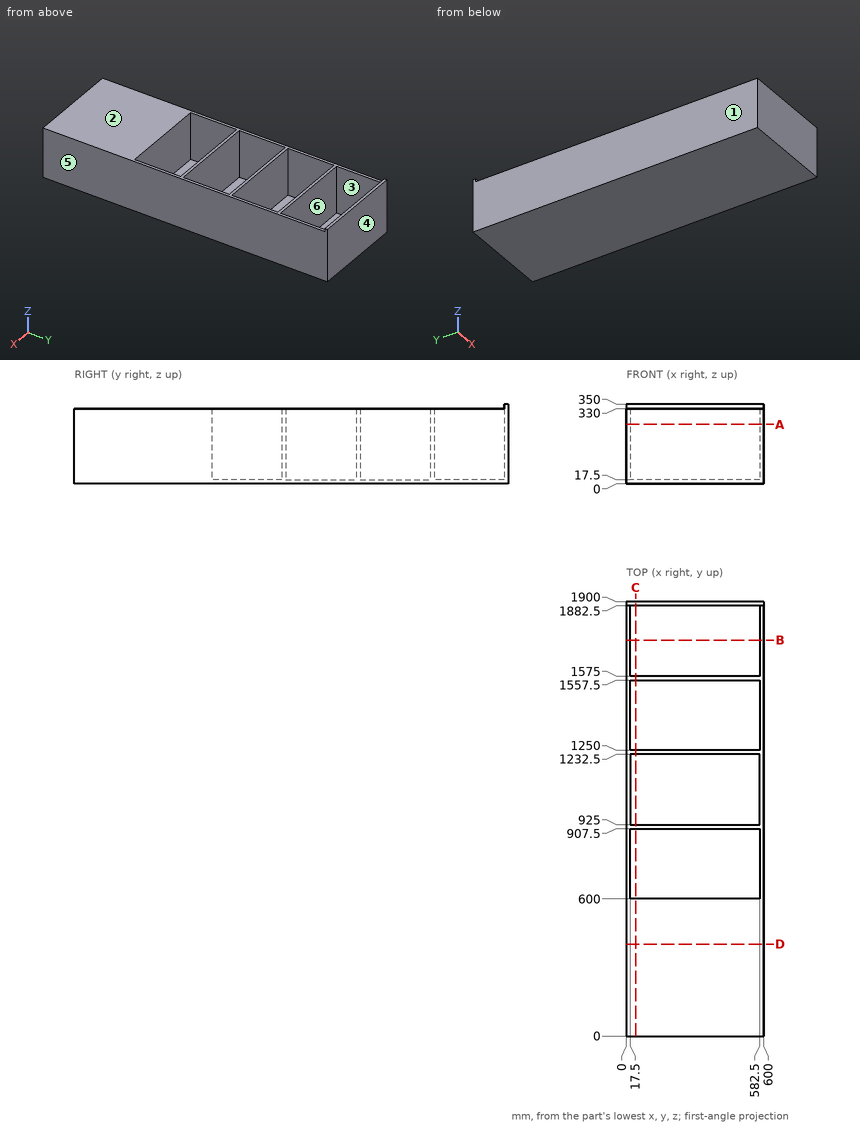
Could you check a few things on this drawing? It's one solid part, dimensions in mm from its lowest x, y, z. A direction names the side the tool comes from. Round coordinates to 2 decimals unless told otherwise and drop trailing zeros. Loops run counter-clockwise (first coordinate to the right, second up) from the corner with the lowest first, then second, coordinate; pieces in that order, holes last. Notation, with made-up numbers: (21.5, 48) -> (76.5, 48) arc R11 cw to (76.5, 59) -> close; hole circle Ø1 at (-30, 63). An arc over 180 degrees is marked (long way). One line per item, written item: value. Start each with the question number.
1. If we section it at C-C, the plane x = 40: Write out the boundary of the cut face in (y, z), then the cut area to 3 significant figures.
2. If we section it at A-A, the plane z = 260.5: Write out the boundary of the cut face in (x, y), then the cut area to 3 significant figures.
3. If we section it at D-D, the plane y = 402: Write out the boundary of the cut face in (x, z), then the cut area to 3 significant figures.
4. For pin 1 (5 mm diameter, centred on x = 304.5, y = 1248, fed in from +Z), with a flat end and sliding along its axis, tell me the tip position at first contact or that it passes through.
5. If I drill on probe 1 along Y at (x, z) = (460.5, 40.5); probe 2 along X at (y, z) = (928, 70.5); probe 3 along Z at (x, y) = (121, 1208), over which ranges is the centre line in solid material (lowest first)?
6. If we mould it in two halves opening along Y, with no side actions, what happens to the marked faces 4, 5 and 6? For each: pulls with the +Y half, pulls with the -Y half, needs draft (parallel to the pull), parting line crosses it, or undercut.
7. If we section it at B-B, the plane y = 1733: Write out the boundary of the cut face in (x, z), then the cut area to 3 significant figures.
8. For the marked faces 1, 2 and 3, which set-ups out of +Z, -Z, +X, -X, +Y, -Y let a thin tool reach every point of the face, with its end or its side?
Calculated:
1. outline: (0, 0) -> (1900, 0) -> (1900, 350) -> (1882.5, 350) -> (1882.5, 17.5) -> (1575, 17.5) -> (1575, 330) -> (1557.5, 330) -> (1557.5, 17.5) -> (1250, 17.5) -> (1250, 330) -> (1232.5, 330) -> (1232.5, 17.5) -> (925, 17.5) -> (925, 330) -> (907.5, 330) -> (907.5, 17.5) -> (600, 17.5) -> (600, 330) -> (0, 330) -> close
1. area: 243,000 mm²
2. outline: (0, 0) -> (600, 0) -> (600, 1900) -> (0, 1900) -> close; hole (17.5, 600) -> (582.5, 600) -> (582.5, 907.5) -> (17.5, 907.5) -> close; hole (17.5, 925) -> (582.5, 925) -> (582.5, 1232.5) -> (17.5, 1232.5) -> close; hole (17.5, 1250) -> (582.5, 1250) -> (582.5, 1557.5) -> (17.5, 1557.5) -> close; hole (17.5, 1575) -> (582.5, 1575) -> (582.5, 1882.5) -> (17.5, 1882.5) -> close
2. area: 445,000 mm²
3. outline: (0, 0) -> (600, 0) -> (600, 330) -> (0, 330) -> close
3. area: 198,000 mm²
4. pin 1: stops at z = 330
5. probe 1: y = 0 to 600, 907.5 to 925, 1232.5 to 1250, 1557.5 to 1575, 1882.5 to 1900
5. probe 2: x = 0 to 17.5, 582.5 to 600
5. probe 3: z = 0 to 17.5
6. face 4: pulls with the +Y half
6. face 5: needs draft
6. face 6: undercut
7. outline: (0, 0) -> (600, 0) -> (600, 330) -> (582.5, 330) -> (582.5, 17.5) -> (17.5, 17.5) -> (17.5, 330) -> (0, 330) -> close
7. area: 21,400 mm²
8. face 1: +Z, -Z, -X, +Y, -Y
8. face 2: +Z, +X, -X, -Y
8. face 3: +Z
